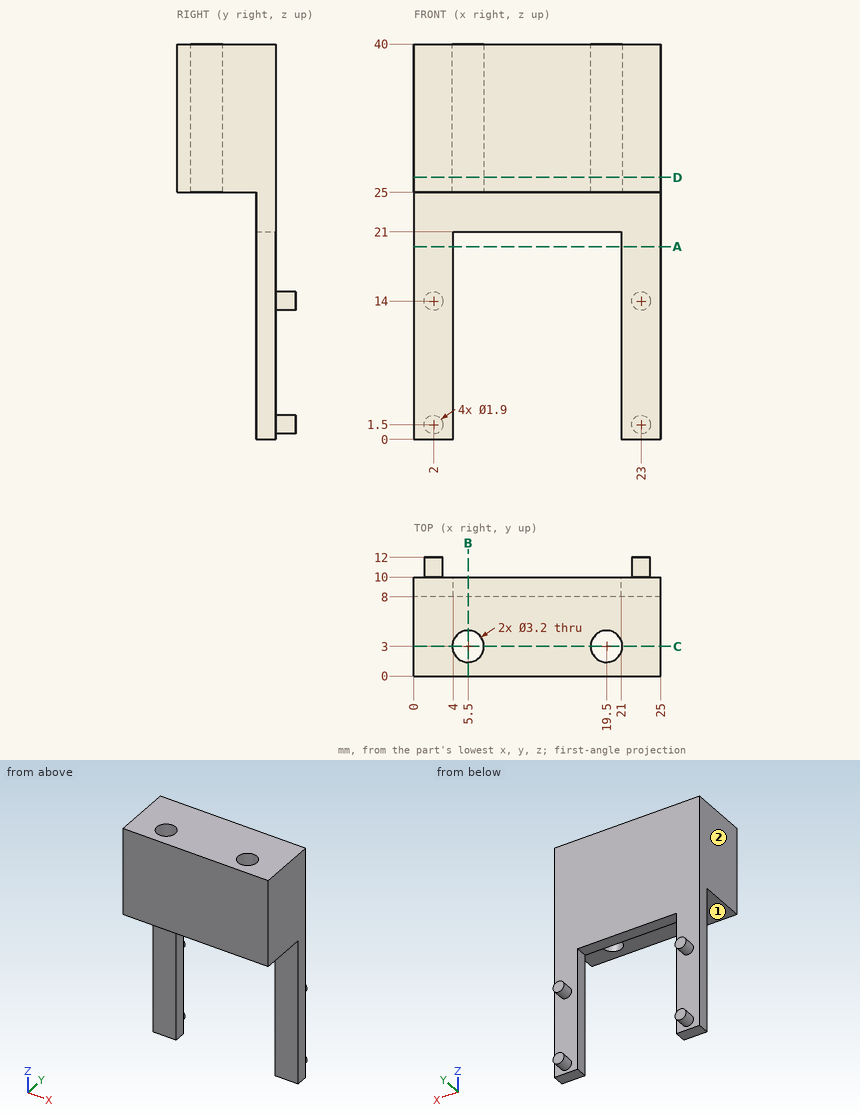
Check sheet for the drawn part. Datum: minimum x, y, z corner. Units: mm. A direction names the side the tool comes from. Give positions to 0.01 mm unless a question says otherwise; leave off trailing zeros. Write each loop counter-clockwise with the first axis right and the second up, starting at its lowest first coordinate (ties: lowest second). Pieces come first, ordered by that corner, then holes. Notation, with made-up numbers: (8.25, -12.5) -> (55.25, -12.5) arc R37 cw to (55.25, 24.5) -> close; hole circle Ø9 at (69.5, 46.25). An arc over 180 degrees is marked (long way). Use one line per item in the form item = value. Start each with the question number.
1. Section check D-D (z = 26.5). Record the cut outline in (x, y).
2. Section check B-B (x = 5.5). Record the cut outline in (y, z), and give its area (3 significant figures).
3. Section check A-A (z = 19.5). Record the cut outline in (x, y), and give its area (3 significant figures).
4. Go/stop test with flat-tipped pins: P1, Ø3.5, axis at x = 5.5, y = 3, coming from the -Z side; P2, Ø1.9, axis at x = 19.5, y = 3, coming from the -Z side; P3, Ø12.5, axis at x = 13.5, z = 16, coming from the +Y side; P4, Ø12, axis at x = 15.5, z = 7, coming from the -Y side. Record where each tip stops, or that it passes through.
5. Access from +Z, -Z, +X, -X, +Y, -Y to the whole of each face (thin tool, end or side, straight path). Record for the marked faces 1 and 2.
6. Thickness scan on line 1 along Y through (x, z) = (5.5, 31.75); line 2 along Z through (x, y) = (17.5, 2); line 3 along Y through (x, z) = (16.25, 27). Record the ranges inside material, lowest first. Write a range as from..to.
7. Section check C-C (y = 3). Record the cut outline in (x, z), and give its area (3 significant figures).
Conclusion:
q1.outline = (0, 0) -> (25, 0) -> (25, 10) -> (0, 10) -> close; hole circle Ø3.2 at (5.5, 3); hole circle Ø3.2 at (19.5, 3)
q2.outline = (0, 25) -> (1.4, 25) -> (1.4, 40) -> (0, 40) -> close; (4.6, 25) -> (8, 25) -> (8, 21) -> (10, 21) -> (10, 40) -> (4.6, 40) -> close
q2.area = 110 mm²
q3.outline = (0, 8) -> (4, 8) -> (4, 10) -> (0, 10) -> close; (21, 8) -> (25, 8) -> (25, 10) -> (21, 10) -> close
q3.area = 16.0 mm²
q4.P1 = 25
q4.P2 = through
q4.P3 = 10
q4.P4 = 8
q5.face_1 = -Z, +X, -X, -Y
q5.face_2 = +Z, -Z, -X, +Y, -Y
q6.line_1 = 0..1.4, 4.6..10
q6.line_2 = 25..40
q6.line_3 = 0..10
q7.outline = (0, 25) -> (3.9, 25) -> (3.9, 40) -> (0, 40) -> close; (7.1, 25) -> (17.9, 25) -> (17.9, 40) -> (7.1, 40) -> close; (21.1, 25) -> (25, 25) -> (25, 40) -> (21.1, 40) -> close
q7.area = 279 mm²
